from build123d import *

# Parameters (mm, degrees)
F0_W     = 365.125
F0_H     = 292.1
F1_DEPTH = 482.6
F2_R     = 25.4
F3_R     = 12.7
F4_T     = -1.5875
F5_R     = 34.925
F6_DEPTH = 365.126
F7_W     = 415.925
F7_H     = 346.075
F8_DEPTH = 88.9
F9_R     = 25.4


with BuildPart() as f1:
    # F0 (on Top) → F1 (new body)
    with BuildSketch(Plane.XY):
        Rectangle(F0_W, F0_H)
    extrude(amount=F1_DEPTH)

    # F2
    f2_edges = [f1.edges().sort_by_distance(p)[0] for p in [
        (-182.5625, -146.05, 241.3),
        (182.5625, -146.05, 241.3),
        (182.5625, 146.05, 241.3),
        (-182.5625, 146.05, 241.3),
    ]]
    fillet(f2_edges, radius=F2_R)

    # F3
    f3_edges = [f1.edges().sort_by_distance(p)[0] for p in [
        (0, -146.05, 0),
    ]]
    fillet(f3_edges, radius=F3_R)

    # F4
    f4_openings = [f1.faces().sort_by_distance(p)[0] for p in [
        (0, 0, 482.6),
    ]]
    offset(amount=F4_T, openings=f4_openings)

    # F5 (on face) → F6 (cut, through all)
    with BuildSketch(Plane.YZ.offset(182.5625)):
        with Locations((0, 225.425)):
            Circle(F5_R)
    extrude(amount=-F6_DEPTH, mode=Mode.SUBTRACT)

    # F7 (on face) → F8 (join)
    with BuildSketch(Plane.XY.offset(482.6)):
        Rectangle(F7_W, F7_H)
        with BuildLine():
            Line((-182.5625, -120.65), (-182.5625, 120.65))
            ThreePointArc((-182.5625, 120.65), (-175.123012, 138.610512), (-157.1625, 146.05))
            Line((-157.1625, 146.05), (157.1625, 146.05))
            ThreePointArc((157.1625, 146.05), (175.123012, 138.610512), (182.5625, 120.65))
            Line((182.5625, 120.65), (182.5625, -120.65))
            ThreePointArc((182.5625, -120.65), (175.123012, -138.610512), (157.1625, -146.05))
            Line((157.1625, -146.05), (-157.1625, -146.05))
            ThreePointArc((-157.1625, -146.05), (-175.123012, -138.610512), (-182.5625, -120.65))
        make_face(mode=Mode.SUBTRACT)
    extrude(amount=-F8_DEPTH)

    # F9
    f9_edges = [f1.edges().sort_by_distance(p)[0] for p in [
        (-207.9625, -173.0375, 438.15),
        (207.9625, -173.0375, 438.15),
        (207.9625, 173.0375, 438.15),
        (-207.9625, 173.0375, 438.15),
    ]]
    fillet(f9_edges, radius=F9_R)


solid = f1.part
Can you work these out from the model? Positions are in its coordinate system, mm. A direction names the side the tool comes from. Round coordinates to 2 decimals unless told otherwise and drop trailing zeros. Write each loop counter-clockwise with the first axis right and the second up, starting at its lowest first coordinate (ties: lowest second). Pieces come first, ordered by that corner, then holes. Notation, with made-up numbers: (44.25, 67.25) -> (75.25, 67.25) arc R23 ccw to (75.25, 92.25) -> close; hole circle Ø3 at (34.5, 4.25). An arc over 180 degrees is marked (long way). Use one line per item in the form item = value. Start each with the question number.
Q1. If I drill on probe 1 along X at (y, z) = (-45, 78) (1 decimal); probe 2 along Y at (x, z) = (120.5, 262); probe 3 along Y at (x, z) = (100.5, 444), over which ranges is the centre line in solid material (lowest first)? Write a range as [from, to].
Q2. Imagine slicing it at D-D (y = 82.5). Please give me the cut outline in (x, z) (1 decimal), then the cut area to 3 significant figures.
Q3. Which directions (+Z, -Z, +X, -X, +Y, -Y) give clear straight access to the entire face, cutting with the end or side of a thin tool? Please do faces 4 (the face through (-2, 146.05, 201)), 5 (the face through (-177.633, -1.689, 4.756)), 6 (the face through (-3, 173.038, 439)).
Q4. We'd pull the mould along X, two halves only. Please class faces 1 (the face through (-2.2, 141.121, 4.756)), 2 (the face through (-207.962, -2, 439)), 3 (the face through (-2, 2, 0)): +X half, -X half, draft (parallel to the pull), parting line (faces both ways), or undercut.
Q5. I'm going to push flat-ended pins straight in: P1, Ø12, axis at x = 103.5, z = 155, coming from the -Y side; P2, Ø12, axis at x = 40.5, z = 331.5, coming from the +Y side; P3, Ø1.5, axis at y = 73.5, z = 380, coming from the -X side. Where does each tip first touch, or does it pass through?
Q6. Imagine slicing it at B-B (y = 0). Count the separate pieces of the cut face and the enclosed holes in it, then the cut area to 3 significant figures.
Worked out:
q1.probe_1 = [-182.6, -181], [181, 182.6]
q1.probe_2 = [-146.05, -144.46], [144.46, 146.05]
q1.probe_3 = [-173.04, -144.46], [144.46, 173.04]
q2.outline = (-208, 393.7) -> (-182.6, 393.7) -> (-182.6, 12.7) arc R12.7 ccw to (-169.9, 0) -> (169.9, 0) arc R12.7 ccw to (182.6, 12.7) -> (182.6, 393.7) -> (208, 393.7) -> (208, 482.6) -> (181, 482.6) -> (181, 12.7) arc R11.1 cw to (169.9, 1.6) -> (-169.9, 1.6) arc R11.1 cw to (-181, 12.7) -> (-181, 482.6) -> (-208, 482.6) -> close
q2.area = 6,610 mm^2
q3.face_4 = -Z, +X, -X, +Y
q3.face_5 = +Z
q3.face_6 = +Z, -Z, +X, -X, +Y
q4.face_1 = undercut
q4.face_2 = -X half
q4.face_3 = draft
q5.P1 = -146.05
q5.P2 = 146.05
q5.P3 = -182.56
q6.separate_pieces = 3
q6.enclosed_holes = 0
q6.area = 6,380 mm^2
